```python
from build123d import *

# Parameters (mm, degrees)
SKETCH1_W           = 203.2
SKETCH1_H           = 63.5
BOSS_EXTRUDE1_DEPTH = 101.6
SKETCH3_W           = 177.8
SKETCH3_H           = 11.43
CUT_EXTRUDE1_DEPTH  = 6.35
CUT_EXTRUDE2_DEPTH  = 11.43
SKETCH5_R           = 6.35
BOSS_EXTRUDE2_DEPTH = 19.05
SKETCH6_R           = 6.858
CUT_EXTRUDE3_DEPTH  = 19.05
SKETCH7_W           = 50.8
SKETCH7_H           = 11.43
CUT_EXTRUDE4_DEPTH  = 161.894515133


with BuildPart() as part:
    # Sketch1 → Boss-Extrude1 (new body)
    with BuildSketch(Plane(origin=(0, 0, 0), x_dir=(1, 0, 0), z_dir=(0, 1, 0))):
        Rectangle(SKETCH1_W, SKETCH1_H)
    extrude(amount=BOSS_EXTRUDE1_DEPTH)

    # Sketch3 → Cut-Extrude1 (cut)
    with BuildSketch(Plane(origin=(0, 101.6, 0), x_dir=(1, 0, 0), z_dir=(0, 1, 0))):
        Rectangle(SKETCH3_W, SKETCH3_H)
    extrude(amount=-CUT_EXTRUDE1_DEPTH, mode=Mode.SUBTRACT)

    # Sketch4 → Cut-Extrude2 (cut)
    with BuildSketch(Plane.XY.offset(-5.715)):
        Polygon((-88.9, 101.6), (-88.9, 57.15), (88.9, 6.35), (88.9, 101.6), align=None)
    extrude(amount=CUT_EXTRUDE2_DEPTH, mode=Mode.SUBTRACT)

    # Sketch5 → Boss-Extrude2 (add)
    with BuildSketch(Plane(origin=(0, 101.6, 0), x_dir=(1, 0, 0), z_dir=(0, 1, 0))):
        with Locations(Location((88.9, -18.7325, 0), (0, 0, 90))):
            Circle(SKETCH5_R)
        with Locations(Location((-88.9, -18.7325, 0), (0, 0, 90))):
            Circle(SKETCH5_R)
        with Locations(Location((-88.9, 18.7325, 0), (0, 0, 90))):
            Circle(SKETCH5_R)
        with Locations(Location((88.9, 18.7325, 0), (0, 0, 90))):
            Circle(SKETCH5_R)
    extrude(amount=BOSS_EXTRUDE2_DEPTH)

    # Sketch6 → Cut-Extrude3 (cut)
    with BuildSketch(Plane.XZ):
        with Locations(Location((88.392, -18.796, 0), (0, 0, 270))):
            Circle(SKETCH6_R)
        with Locations(Location((-88.392, -18.796, 0), (0, 0, 270))):
            Circle(SKETCH6_R)
        with Locations(Location((-88.392, 18.669, 0), (0, 0, 270))):
            Circle(SKETCH6_R)
        with Locations(Location((88.392, 18.669, 0), (0, 0, 270))):
            Circle(SKETCH6_R)
    extrude(amount=-CUT_EXTRUDE3_DEPTH, mode=Mode.SUBTRACT)

    # Sketch7 → Cut-Extrude4 (cut, through all)
    with BuildSketch(Plane.XZ):
        with Locations((63.5, 0)):
            Rectangle(SKETCH7_W, SKETCH7_H)
    extrude(amount=-CUT_EXTRUDE4_DEPTH, mode=Mode.SUBTRACT)


solid = part.part
```
CAD build for the part. Positions are in the model's coordinates, mm. A direction names the side the tool comes from. Give positions to 0.01 mm unless a question says otherwise; leave off trailing zeros. Write each loop counter-clockwise with the first axis right and the second up, starting at its lowest first coordinate (ties: lowest second). Pieces come first, ordered by that corner, then holes. Notation, with made-up numbers: M -5,53.25 L 4,53.25 A22 ccw 4,75.25 Z; hole C -14,-39 d10. An arc over 180 degrees is marked long. Return JSON: item names as keys, results as strings. Group by question number.
(1) Band-saw the part on B-B (z = 2). Give the cut face in (x, y), and give its area (3 significant figures).
(2) 3-axis set-ups, long thin cutter, end or side, ignore diameter. For faces 4 (the face through (-88, 19.05, 19)), 5 (the face through (19, 61, 5.715)), 6 (the face through (88.9, 50, 0)): which of +Z, -Z, +X, -X, +Y, -Y reach the whole face in a straight line?
(3) Band-saw the part on C-C (y = 85). Give the cut face in (x, z) (3 decimals).
(4) Band-saw the part on D-D (z = -8.5). Give the cut face in (x, y).
(5) Flat gauge pin, fed straight in: pin 1 Ø8 at (x, z) = (88.392, 18.669) entering from -Y. Where does the tip first touch, or does it go through?
(6) Mould opens along X. For faces 1 (the face through (101.6, 50, 0)), 2 (the face through (89, 120.65, 19)), 3 (the face through (19, 61, -5.715)) say: pulls with the +X half, pulls with the -X half, needs draft (parallel to the pull), parting line crosses it, or undercut.
(7) Band-saw the part on A-A (x = 64). Give the cut face in (y, z) (3 decimals), and give its area (3 significant figures).
(8) Drill centre lines: L1, parallel to Z at x = 47, y = 52.5 (3 decimals); L2, parallel to Y at x = 41, z = 16; L3, parallel to X at y = 110, z = -22. Where is each one in solid material? Low to high. Write a range as [from, to].
Entries:
{
 "1": {"outline": "M -101.6,0 L 38.1,0 L 38.1,20.86 L -88.9,57.15 L -88.9,101.6 L -101.6,101.6 Z; M 88.9,0 L 101.6,0 L 101.6,101.6 L 88.9,101.6 Z", "area": "7,530 mm^2"},
 "2": {"face 4": "-Y", "face 5": "+Y", "face 6": "+Y, -Y"},
 "3": {"outline": "M -101.6,-31.75 L 101.6,-31.75 L 101.6,31.75 L -101.6,31.75 Z; hole M -88.9,-5.715 L 88.9,-5.715 L 88.9,5.715 L -88.9,5.715 Z"},
 "4": {"outline": "M -101.6,0 L 101.6,0 L 101.6,101.6 L -101.6,101.6 Z"},
 "5": {"pin 1": "stops at y = 19.05"},
 "6": {"face 1": "pulls with the +X half", "face 2": "needs draft", "face 3": "undercut"},
 "7": {"outline": "M 0,-31.75 L 101.6,-31.75 L 101.6,-5.715 L 0,-5.715 Z; M 0,5.715 L 101.6,5.715 L 101.6,31.75 L 0,31.75 Z", "area": "5,290 mm^2"},
 "8": {"L1": "z = [-31.75, -5.715], [5.715, 31.75]", "L2": "y = [0, 101.6]", "L3": "x = [-94.34, -83.46], [83.46, 94.34]"}
}
